The model under review builds one solid part; all positions refer to its coordinate system, in mm. Face numbers are marked on the shaded views. A direction names the side the tool comes from. Round coordinates to 2 decimals unless told otherwise and drop trailing zeros. Write each loop counter-clockwise with the first axis right and the second up, starting at its lowest first coordinate (ties: lowest second). Pieces come first, ordered by that corner, then holes. Notation, with made-up numbers: (59, -21) -> (103, -21) arc R6 cw to (103, -12) -> close; hole circle Ø6 at (27.5, 19). An arc over 180 degrees is marked (long way). Answer as a JSON object with one key per item and string values. Group by question number.
1) We need section D-D, the plane y = 10.5. Write out the cut boundary in (x, z).
2) Mouldability with a two-part tool opening along X and no side actions: class the marked faces 4, 5 and 6 as pulls with the +X half, pulls with the -X half, needs draft (parallel to the pull), parting line crosses it, or undercut.
3) We need section C-C, the plane z = 12. Write out the cut boundary in (x, y).
4) To check wall thickness, follow probe 1 along Y at (x, z) = (57.75, 12); probe 2 along Y at (x, z) = (0.5, -0.5); probe 3 along Z at (x, y) = (24, 24). State the ranges of each line that lie inside material, in increasing order. Write a range as [from, to].
5) Machinability: for the marked faces 1, 2 and 3, which of the approach directions +Z, -Z, +X, -X, +Y, -Y give a long, thin tool a straight path to every point of the face, cutting with its end or side? Answer none if there is none.
6) Insertion check: pin 1 Ø16.5 at (y, z) = (5.5, 9) entering from +X; pin 2 Ø1.2 at (x, z) = (61, 11.5) entering from -Y; pin 3 Ø6 at (x, y) = (46, 15.5) entering from -Z; pin 4 Ø2.5 at (y, z) = (20, -15) entering from -X. Each pin has a flat end and moves straight along its axis. Give the tip position at first contact, or say it passes through.
7) We need section A-A, the plane z = -15. Write out the cut boundary in (x, y).
8) We need section B-B, the plane x = 59. Write out the cut boundary in (y, z).
from build123d import *

# Parameters (mm, degrees)
SKETCH1_W           = 10
SKETCH1_H           = 60
BOSS_EXTRUDE1_DEPTH = 15
SKETCH4_W           = 10
SKETCH4_H           = 15
BOSS_EXTRUDE2_DEPTH = 60
BOSS_EXTRUDE4_DEPTH = 10
SKETCH6_R           = 2
CUT_EXTRUDE1_DEPTH  = 10
SKETCH7_R           = 2
BOSS_EXTRUDE6_DEPTH = 10


with BuildPart() as part:
    # Sketch1 → Boss-Extrude1 (new body)
    with BuildSketch(Plane.XY):
        Rectangle(SKETCH1_W, SKETCH1_H)
    extrude(amount=BOSS_EXTRUDE1_DEPTH)

    # Sketch4 → Boss-Extrude2 (add)
    with BuildSketch(Plane(origin=(5, 0, 0), x_dir=(0, 0, -1), z_dir=(1, 0, 0))):
        with Locations((-5, 22.5)):
            Rectangle(SKETCH4_W, SKETCH4_H)
    extrude(amount=BOSS_EXTRUDE2_DEPTH)

    # Sketch5 → Boss-Extrude4 (add)
    # profile 1 of 5: a face of its own
    with BuildSketch(Plane(origin=(65, 0, 0), x_dir=(0, 0, -1), z_dir=(1, 0, 0))):
        with BuildLine():
            Line((-10, 20), (-10, 23))
            Line((-10, 23), (-14, 23))
            ThreePointArc((-14, 23), (-15.060660172, 22.560660172), (-15.5, 21.5))
            Line((-15.5, 21.5), (-15.5, 18.5))
            ThreePointArc((-15.5, 18.5), (-15.060660172, 17.439339828), (-14, 17))
            Line((-14, 17), (-10, 17))
            Line((-10, 17), (-10, 20))
        make_face()
        with BuildLine():
            ThreePointArc((-14, 20), (-12, 22), (-10, 20))
            ThreePointArc((-10, 20), (-12, 18), (-14, 20))
        make_face(mode=Mode.SUBTRACT)
    # profile 2 of 5: a face of its own
    with BuildSketch(Plane(origin=(65, 0, 0), x_dir=(0, 0, -1), z_dir=(1, 0, 0))):
        with BuildLine():
            ThreePointArc((-14, 20), (-12, 18), (-10, 20))
            Line((-10, 20), (-12, 20))
            Line((-12, 20), (-14, 20))
        make_face()
    # profile 3 of 5: a face of its own
    with BuildSketch(Plane(origin=(65, 0, 0), x_dir=(0, 0, -1), z_dir=(1, 0, 0))):
        with BuildLine():
            Line((-12, 20), (-10, 20))
            ThreePointArc((-10, 20), (-12, 22), (-14, 20))
            Line((-14, 20), (-12, 20))
        make_face()
    # profile 4 of 5: a face of its own
    with BuildSketch(Plane(origin=(65, 0, 0), x_dir=(0, 0, -1), z_dir=(1, 0, 0))):
        with BuildLine():
            ThreePointArc((-14, 20), (-12, 18), (-10, 20))
            Line((-10, 20), (-12, 20))
            Line((-12, 20), (-14, 20))
        make_face()
    # profile 5 of 5: a face of its own
    with BuildSketch(Plane(origin=(65, 0, 0), x_dir=(0, 0, -1), z_dir=(1, 0, 0))):
        with BuildLine():
            Line((-12, 20), (-10, 20))
            ThreePointArc((-10, 20), (-12, 22), (-14, 20))
            Line((-14, 20), (-12, 20))
        make_face()
    extrude(amount=-BOSS_EXTRUDE4_DEPTH)

    # Sketch6 → Cut-Extrude1 (cut)
    with BuildSketch(Plane(origin=(65, 0, 0), x_dir=(0, 0, -1), z_dir=(1, 0, 0))):
        with Locations((-12, 20)):
            Circle(SKETCH6_R)
    extrude(amount=-CUT_EXTRUDE1_DEPTH, mode=Mode.SUBTRACT)

    # Sketch7 → Boss-Extrude6 (add)
    with BuildSketch(Plane(origin=(-5, 0, 0), x_dir=(0, 0, -1), z_dir=(1, 0, 0))):
        with BuildLine():
            Line((10, 23), (0, 23))
            Line((0, 23), (0, 17))
            Line((0, 17), (10, 17))
            Line((10, 17), (17, 17))
            ThreePointArc((17, 17), (18.060660172, 17.439339828), (18.5, 18.5))
            Line((18.5, 18.5), (18.5, 21.5))
            ThreePointArc((18.5, 21.5), (18.060660172, 22.560660172), (17, 23))
            Line((17, 23), (10, 23))
        make_face()
        with Locations((15, 20)):
            Circle(SKETCH7_R, mode=Mode.SUBTRACT)
    extrude(amount=BOSS_EXTRUDE6_DEPTH)


solid = part.part
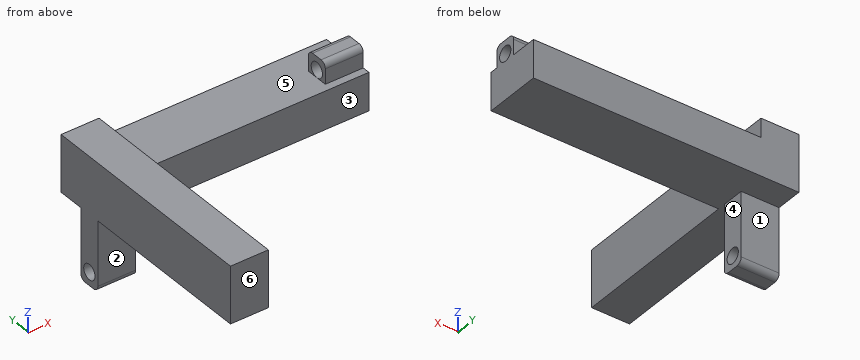
Here are the results:
{
 "1": {"outline": "(-5, 0) -> (5, 0) -> (5, 15) -> (-5, 15) -> close"},
 "2": {"face 4": "pulls with the +X half", "face 5": "undercut", "face 6": "needs draft"},
 "3": {"outline": "(-5, -30) -> (5, -30) -> (5, 30) -> (-5, 30) -> close; (55, 17) -> (65, 17) -> (65, 18) -> (55, 18) -> close; (55, 22) -> (65, 22) -> (65, 23) -> (55, 23) -> close"},
 "4": {"probe 1": "y = [17, 18], [22, 23]", "probe 2": "y = [17, 23]", "probe 3": "z = [0, 10]"},
 "5": {"face 1": "-Z, +X, -X, +Y", "face 2": "-Z, +X, -X, -Y", "face 3": "+Z, -Z, +X, -Y"},
 "6": {"pin 1": "stops at x = 5", "pin 2": "stops at y = 17", "pin 3": "stops at z = 0", "pin 4": "passes through"},
 "7": {"outline": "(-5, 17) -> (5, 17) -> (5, 18) -> (-5, 18) -> close; (-5, 22) -> (5, 22) -> (5, 23) -> (-5, 23) -> close"},
 "8": {"outline": "(15, 0) -> (30, 0) -> (30, 10) -> (23, 10) -> (23, 14) arc R1.5 ccw to (21.5, 15.5) -> (18.5, 15.5) arc R1.5 ccw to (17, 14) -> (17, 10) -> (15, 10) -> close; hole circle Ø4 at (20, 12)"}
}
